Work out the finished part from the listing and answer in its coordinate system (mm). A direction names the side the tool comes from. Give positions to 0.01 mm unless a question says otherwise; leave off trailing zeros. Loops run counter-clockwise (first coordinate to the right, second up) from the corner with the lowest first, then second, coordinate; pieces in that order, holes last.
from build123d import *

# Parameters (mm, degrees)
SKETCH_1_R                = 51.5
EXTRUDE_1_DEPTH           = 45
CUT_EXTRUDE_1_DEPTH       = 86.612499087
CUT_EXTRUDE_1_DEPTH_BACK  = 86.612499087
FILLET_1_R                = 3
HOLE_WIZARD_1_D           = 1.8
HOLE_WIZARD_1_CBORE_D     = 3.3
HOLE_WIZARD_1_CBORE_DEPTH = 1.8
PATTERN_CIRCULAR_1_COUNT  = 4
SHELL_START               = 3
SHELL_5_DEPTH             = 40.851543255
SHELL_START_2             = 4.8
SHELL_5_2_DEPTH           = 39.051543255


# Read off the part's stored shape, not the designer's step: 抽壳5
with BuildPart() as part:
    # 草图1 → 凸台-拉伸1 (new body)
    with BuildSketch(Plane.XY):
        with Locations(Location((0, 0, 0), (0, 0, 180))):
            Circle(SKETCH_1_R)
    extrude(amount=EXTRUDE_1_DEPTH)

    # 草图2 → 切除-拉伸1 (cut, two sides: drawn at the far end of the back side and taken through both)
    with BuildSketch(Plane(origin=(0, 0, 0), x_dir=(1, 0, 0), z_dir=(0, 1, 0)).offset(-CUT_EXTRUDE_1_DEPTH_BACK)):
        Polygon((-51.5, -45), (51.5, -45), (51.5, -7.511065871), align=None)
    extrude(amount=CUT_EXTRUDE_1_DEPTH + CUT_EXTRUDE_1_DEPTH_BACK, mode=Mode.SUBTRACT)

    # 圆角1
    fillet_1_edges = [part.edges().sort_by_distance(p)[0] for p in [
        (51.5, 0, 0),
    ]]
    fillet(fillet_1_edges, radius=FILLET_1_R)

    # 打孔尺寸(%根据)内六角圆柱头螺钉的类型1 (through all)
    with Locations(Plane(origin=(0, 0, 0), x_dir=(-1, 0, 0), z_dir=(0, 0, -1))):
        with Locations((0, 48.75)):
            hole_wizard_1 = CounterBoreHole(HOLE_WIZARD_1_D / 2, HOLE_WIZARD_1_CBORE_D / 2, HOLE_WIZARD_1_CBORE_DEPTH)

    # 阵列(圆周)1: 打孔尺寸(%根据)内六角圆柱头螺钉的类型1 ×4 about axis
    pattern_circular_1_axis = Axis((0, 0, 0), (0, 0, 1))
    for i in range(1, PATTERN_CIRCULAR_1_COUNT):
        add(hole_wizard_1.rotate(pattern_circular_1_axis, i * 360 / PATTERN_CIRCULAR_1_COUNT), mode=Mode.SUBTRACT)

    # 抽壳5 outline → 抽壳5 (cut)
    with BuildSketch(Plane.XY.offset(SHELL_START)):
        with BuildLine():
            ThreePointArc((-48.278871795, -4.626071575), (-34.294678888, -34.294678888), (-4.626071575, -48.278871795))
            ThreePointArc((-4.626071575, -48.278871795), (0, -44.1), (4.626071575, -48.278871795))
            ThreePointArc((4.626071575, -48.278871795), (34.294678888, -34.294678888), (48.278871795, -4.626071575))
            ThreePointArc((48.278871795, -4.626071575), (44.1, 0), (48.278871795, 4.626071575))
            ThreePointArc((48.278871795, 4.626071575), (34.294678888, 34.294678888), (4.626071575, 48.278871795))
            ThreePointArc((4.626071575, 48.278871795), (0, 44.1), (-4.626071575, 48.278871795))
            ThreePointArc((-4.626071575, 48.278871795), (-34.294678888, 34.294678888), (-48.278871795, 4.626071575))
            ThreePointArc((-48.278871795, 4.626071575), (-44.1, 0), (-48.278871795, -4.626071575))
        make_face()
    extrude(amount=SHELL_5_DEPTH, mode=Mode.SUBTRACT)

    # Shell 5 2 outline → Shell 5 2 (cut)
    with BuildSketch(Plane.XY.offset(SHELL_START_2)):
        with BuildLine():
            ThreePointArc((4.626071575, -48.278871795), (0, -44.1), (-4.626071575, -48.278871795))
            ThreePointArc((-4.626071575, -48.278871795), (-4.252601262, -48.313200914), (-3.878876655, -48.344641026))
            ThreePointArc((-3.878876655, -48.344641026), (0, -44.85), (3.878876655, -48.344641026))
            ThreePointArc((3.878876655, -48.344641026), (4.252601262, -48.313200914), (4.626071575, -48.278871795))
        make_face()
        with BuildLine():
            ThreePointArc((-48.344641026, -3.878876655), (-48.313200914, -4.252601262), (-48.278871795, -4.626071575))
            ThreePointArc((-48.278871795, -4.626071575), (-44.1, 0), (-48.278871795, 4.626071575))
            ThreePointArc((-48.278871795, 4.626071575), (-48.313200914, 4.252601262), (-48.344641026, 3.878876655))
            ThreePointArc((-48.344641026, 3.878876655), (-44.85, 0), (-48.344641026, -3.878876655))
        make_face()
        with BuildLine():
            ThreePointArc((48.278871795, 4.626071575), (44.1, 0), (48.278871795, -4.626071575))
            ThreePointArc((48.278871795, -4.626071575), (48.313200914, -4.252601262), (48.344641026, -3.878876655))
            ThreePointArc((48.344641026, -3.878876655), (44.85, 0), (48.344641026, 3.878876655))
            ThreePointArc((48.344641026, 3.878876655), (48.313200914, 4.252601262), (48.278871795, 4.626071575))
        make_face()
        with BuildLine():
            ThreePointArc((-3.878876655, 48.344641026), (-4.252601262, 48.313200914), (-4.626071575, 48.278871795))
            ThreePointArc((-4.626071575, 48.278871795), (0, 44.1), (4.626071575, 48.278871795))
            ThreePointArc((4.626071575, 48.278871795), (4.252601262, 48.313200914), (3.878876655, 48.344641026))
            ThreePointArc((3.878876655, 48.344641026), (0, 44.85), (-3.878876655, 48.344641026))
        make_face()
    extrude(amount=SHELL_5_2_DEPTH, mode=Mode.SUBTRACT)


solid = part.part
Item 1: Flat-ended cylindrical pins translate along their axes: pin 1 Ø3 at (x, y) = (48.75, 0) entering from -Z; pin 2 Ø12 at (x, y) = (-12.5, -17.5) entering from -Z; pin 3 Ø2 at (x, y) = (-45.5, 0) entering from +Z; pin 4 Ø8 at (x, z) = (-7.5, 29.5) entering from -Y. Find the tip coordinate at first contact, or state that the pin passes through.
Item 2: For faces 1 (the face through (-0.36, -47.14, 0.89)), 2 (the face through (44.6, 0, 4.8)), determine the directions among +Z, -Z, +X, -X, +Y, -Y from which every point of the face is accessible in a straight line to the end or side of a thin tool.
Item 3: Find section B-B, the plane z = 13. Write down the section's boundary in (x, y).
Item 4: Consider line 1 (Y direction, x = 0, z = 1.2); line 2 (Y direction, x = -36, z = 8); line 3 (Z direction, x = -25.5, y = 12.5). Determine where each line is inside the solid, lowest interval first.
Item 5: Find section A-A, the plane z = 40. Write down the section's boundary in (x, y), plus the area to 3 significant figures.
Item 6: Determine the mould class of faces 3 (the face through (-49.12, -15.47, 19.04)), 4 (the face through (0.36, 47.14, 0.89)), 5 (the face through (0.24, -46.02, 26.17)) for opening direction X: released by +X, released by -X, zero draft, split by the parting line, or undercut.
Ans:
1. pin 1: stops at z = 1.8
1. pin 2: stops at z = 0
1. pin 3: stops at z = 43.18
1. pin 4: stops at y = -51.35
2. face 1: -Z
2. face 2: +Z
3. outline: (-48.34, -3.88) arc R3.9 ccw to (-48.34, 3.88) arc R48.5 cw to (-48.28, 4.63) arc R48.5 cw to (-4.63, 48.28) arc R48.5 cw to (-3.88, 48.34) arc R3.9 ccw to (3.88, 48.34) arc R48.5 cw to (4.63, 48.28) arc R48.5 cw to (36.42, 32.03) - (36.42, 36.41) arc R51.5 ccw (long way) to (36.42, -36.41) - (36.42, -32.03) arc R48.5 cw to (4.63, -48.28) arc R48.5 cw to (3.88, -48.34) arc R3.9 ccw to (-3.88, -48.34) arc R48.5 cw to (-4.63, -48.28) arc R48.5 cw to (-48.28, -4.63) arc R48.5 cw to start; hole circle Ø1.8 at (-48.75, 0); hole circle Ø1.8 at (0, -48.75); hole circle Ø1.8 at (0, 48.75)
4. line 1: y = -50.9 to -50.4, -47.1 to 47.1, 50.4 to 50.9
4. line 2: y = -36.83 to -32.5, 32.5 to 36.83
4. line 3: z = 0 to 3
5. outline: (-48.34, -3.88) arc R3.9 ccw to (-48.34, 3.88) arc R48.5 cw to (-48.28, 4.63) arc R48.5 cw to (-37.76, 30.43) - (-37.76, 35.02) arc R51.5 ccw to (-37.76, -35.02) - (-37.76, -30.43) arc R48.5 cw to (-48.28, -4.63) arc R48.5 cw to start; hole circle Ø1.8 at (-48.75, 0)
5. area: 233 mm2
6. face 3: split by the parting line
6. face 4: undercut
6. face 5: released by +X
